Solid Edge part; units mm, degrees
sketch "Sketch1" plane through (0, 0, 0) normal (0, 0, 1) x (1, 0, 0)
  line L0 (10, -10) -> (-10, -10)
  line L1 (-10, -10) -> (-10, 10)
  line L2 (-10, 10) -> (10, 10)
  line L3 (10, 10) -> (10, -10)
  circle A0 centre (0, 0) radius 2.5
extrude "Protrusion1" add sketch "Sketch1" along normal blind 5
fillet "Round_1" radius 5 4 edges at (10, -10, 2.5) (10, 10, 2.5) (-10, 10, 2.5) (-10, -10, 2.5)
sketch "Sketch2" plane through (0, 0, 0) normal (1, 0, 0) x (0, 1, 0)
  line L0 (-10, 5) -> (-7.5, 5)
  line L1 (-7.5, 14.5) -> (-7.5, 5)
  line L2 (7.5, 14.5) -> (7.5, 5)
  line L3 (7.5, 5) -> (10, 5)
  line L4 (10, 5) -> (10, 22)
  arc A0 (7, 25) -> (10, 22) centre (7, 22) cw
  line L5 (7, 25) -> (-7, 25)
  arc A1 (-7, 25) -> (-10, 22) centre (-7, 22) ccw
  line L6 (-10, 22) -> (-10, 5)
  arc A2 (-7.5, 14.5) -> (7.5, 14.5) centre (0, 14.5) cw
extrude "ExtrudedProtrusion_2" add sketch "Sketch2" along normal mid plane 6
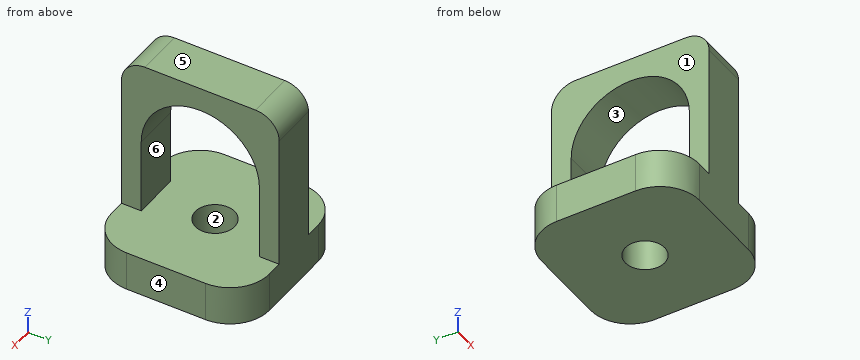
Input: part model. Units: mm. Frame: model coordinates. Face numbers are marked on the shaded views. A direction names the side the tool comes from. Coordinates: 2 decimals unless noted, no trailing zeros. Loops run counter-clockwise (first coordinate to the right, second up) from the corner with the lowest first, then second, coordinate; pieces in that order, holes last. Notation, with made-up numbers: M -26.75,42 L -5.75,42 A20 ccw -5.75,48 Z; hole C -30.5,70.25 d2. An arc over 180 degrees is marked long. Use a Markdown table: item, result. Add a question column.
1) Pin query (flat end, axial travel): P1, Ø6, axis at y = 4, z = 10.5, coming from the -X side; P2, Ø3, axis at y = -6, z = 22.5, coming from the -X side. Return the tip coordinate at first contact, or that it passes through.
2) Section A-A, the plane z = 10. Return the cut outline in (x, y), plus the area to 3 significant figures.
3) Line query: L1, parallel to Y at x = 0, z = 12.75; L2, parallel to Y at x = 0, z = 2.05; L3, parallel to Z at x = 7.75, y = -4.75. Output: solid intervals per line, ascending. Write a range as from..to.
4) Section B-B, the plane y = 4. Return the cut outline in (x, z).
5) Draft query along Z for the marked faces 4, 5 and 6. Return one class per face: +Z half, -Z half, draft (parallel to the pull), parting line (faces both ways), or undercut.
6) Set-up query: the marked faces 1, 2 and 3. Return all of +Z, -Z, +X, -X, +Y, -Y with unobstructed straight access to the full face (end or side cutting, diameter ignored); none if empty.
7) Section D-D, the plane x = 0. Return the cut outline in (y, z), plus the area to 3 significant figures.
8) Section C-C, the plane y = 0. Return the cut outline in (x, z), plus the area to 3 significant figures.
Answer below:
| question | item | result |
|---|---|---|
| 1 | P1 | through |
| 1 | P2 | x = -3 |
| 2 | outline | M -3,-10 L 3,-10 L 3,-7.5 L -3,-7.5 Z; M -3,7.5 L 3,7.5 L 3,10 L -3,10 Z |
| 2 | area | 30.0 mm2 |
| 3 | L1 | -10..-7.5, 7.5..10 |
| 3 | L2 | -10..-2.5, 2.5..10 |
| 3 | L3 | 0..5 |
| 4 | outline | M -10,0 L 10,0 L 10,5 L -10,5 Z; M -3,20.84 L 3,20.84 L 3,25 L -3,25 Z |
| 5 | face 4 | draft |
| 5 | face 5 | +Z half |
| 5 | face 6 | undercut |
| 6 | face 1 | +Z, -X, +Y, -Y |
| 6 | face 2 | -Z |
| 6 | face 3 | +X, -X |
| 7 | outline | M -10,0 L -2.5,0 L -2.5,5 L -7.5,5 L -7.5,14.5 A7.5 cw 7.5,14.5 L 7.5,5 L 2.5,5 L 2.5,0 L 10,0 L 10,22 A3 ccw 7,25 L -7,25 A3 ccw -10,22 Z |
| 7 | area | 240 mm2 |
| 8 | outline | M -10,0 L -2.5,0 L -2.5,5 L -10,5 Z; M -3,22 L 3,22 L 3,25 L -3,25 Z; M 2.5,0 L 10,0 L 10,5 L 2.5,5 Z |
| 8 | area | 93.0 mm2 |
